Read the model definition and answer for the solid it produces. Units are mm, in the model's axes. Face numbers are marked on the shaded views. A direction names the side the tool comes from. Round coordinates to 2 decimals unless told otherwise and drop trailing zeros. Order: outer loops, then holes, each group sorted by start corner. A loop starts at its lowest first (then second) coordinate and runs counter-clockwise, first axis right, second up. Notation, with made-up numbers: (43, 64.25) - (56, 64.25) arc R16 ccw to (56, 76.25) - close; hole circle Ø8 at (85.25, 3). An arc over 180 degrees is marked (long way). One line per question, with ' | ' between items. Start each with the question number.
1) The part is cut by section A-A, the plane z = 9. Give the vertices of the cut face in (x, y), plus the area to 3 significant figures.
2) Straight lines are drawn through the part: line 1 (Y direction, x = 32, z = 6.5); line 2 (Y direction, x = 38.75, z = 1.05). For each, find the intervals that lie inside material, in ascending order. Write a range as from..to.
3) The part is cut by section C-C, the plane z = 16. Give the vertices of the cut face in (x, y), plus the area to 3 significant figures.
4) For the marked faces 4, 5 and 6, determine the directions among +Z, -Z, +X, -X, +Y, -Y from which every point of the face is accessible in a straight line to the end or side of a thin tool.
5) The part is cut by section D-D, the plane x = 23.3. Give the vertices of the cut face in (y, z).
6) Flat-ended cylindrical pins translate along their axes: pin 1 (1.6 mm diameter, centred on y = 1, z = 13.5, fed in from +X); pin 2 (1.8 mm diameter, centred on x = 38.75, y = 38.75, fed in from +Z); pin 3 (3.5 mm diameter, centred on x = 38.75, y = 7.75, fed in from +Z); pin 4 (2 mm diameter, centred on x = 45.5, z = 13, fed in from +Y). Find the tip coordinate at first contact, or state that the pin passes through.
7) The part is cut by section B-B, the plane y = 23.3. Give the vertices of the cut face in (x, z), plus the area to 3 significant figures.
8) The mould has two halves that part along Y. Classify the marked faces 1, 2 and 3: pulls with the +Y half, pulls with the -Y half, needs draft (parallel to the pull), parting line crosses it, or undercut.
from build123d import *

# Parameters (mm, degrees)
F0_W      = 46.5
F0_H      = 46.5
F0_R      = 1.5
F0_R_2    = 17.5
F1_DEPTH  = 3
F2_W      = 42.5
F2_H      = 2
F3_DEPTH  = 15
F4_W      = 10
F4_H      = 15
F5_DEPTH  = 10
F6_W      = 10
F6_H      = 15
F7_DEPTH  = 10
F8_W      = 10
F8_H      = 15
F9_DEPTH  = 10
F10_W     = 10
F10_H     = 15
F11_DEPTH = 10
F12_R     = 5
F13_R     = 5
F14_R     = 5
F15_R     = 5
F16_W     = 10
F16_H     = 8
F17_DEPTH = 25
F18_R     = 1
F19_R     = 1


with BuildPart() as f1:
    # F0 (on Top) → F1 (new body)
    with BuildSketch(Plane.XY):
        with Locations((23.25, 23.25)):
            Rectangle(F0_W, F0_H)
        with Locations((7.75, 7.75)):
            Circle(F0_R, mode=Mode.SUBTRACT)
        with Locations((38.75, 7.75)):
            Circle(F0_R, mode=Mode.SUBTRACT)
        with Locations((7.75, 38.75)):
            Circle(F0_R, mode=Mode.SUBTRACT)
        with Locations((23.3, 23.3)):
            Circle(F0_R_2, mode=Mode.SUBTRACT)
        with Locations((38.75, 38.75)):
            Circle(F0_R, mode=Mode.SUBTRACT)
    extrude(amount=F1_DEPTH)

    # F2 (on face) → F3 (join)
    with BuildSketch(Plane.XY.offset(3)):
        Polygon((2, 46.5), (0, 46.5), (0, 0), (2, 0), (2, 2), (2, 44.5), align=None)
        with Locations((23.25, 45.5)):
            Rectangle(F2_W, F2_H)
        Polygon((46.5, 46.5), (44.5, 46.5), (44.5, 44.5), (44.5, 2), (44.5, 0), (46.5, 0), align=None)
        with Locations((23.25, 1)):
            Rectangle(F2_W, F2_H)
    extrude(amount=F3_DEPTH)

    # F4 (on face) → F5 (cut)
    with BuildSketch(Plane.XZ):
        with Locations((5, 10.5)):
            Rectangle(F4_W, F4_H)
    extrude(amount=-F5_DEPTH, mode=Mode.SUBTRACT)

    # F6 (on face) → F7 (cut)
    with BuildSketch(Plane(origin=(0, 46.5, 0), x_dir=(-1, 0, 0), z_dir=(0, 1, 0))):
        with Locations((-5, 10.5)):
            Rectangle(F6_W, F6_H)
    extrude(amount=-F7_DEPTH, mode=Mode.SUBTRACT)

    # F8 (on face) → F9 (cut)
    with BuildSketch(Plane(origin=(0, 46.5, 0), x_dir=(-1, 0, 0), z_dir=(0, 1, 0))):
        with Locations((-41.5, 10.5)):
            Rectangle(F8_W, F8_H)
    extrude(amount=-F9_DEPTH, mode=Mode.SUBTRACT)

    # F10 (on face) → F11 (cut)
    with BuildSketch(Plane.XZ):
        with Locations((41.5, 10.5)):
            Rectangle(F10_W, F10_H)
    extrude(amount=-F11_DEPTH, mode=Mode.SUBTRACT)

    # F12
    f12_edges = [f1.edges().sort_by_distance(p)[0] for p in [
        (46.5, 46.5, 1.5),
    ]]
    fillet(f12_edges, radius=F12_R)

    # F13
    f13_edges = [f1.edges().sort_by_distance(p)[0] for p in [
        (0, 46.5, 1.5),
    ]]
    fillet(f13_edges, radius=F13_R)

    # F14
    f14_edges = [f1.edges().sort_by_distance(p)[0] for p in [
        (46.5, 0, 1.5),
    ]]
    fillet(f14_edges, radius=F14_R)

    # F15
    f15_edges = [f1.edges().sort_by_distance(p)[0] for p in [
        (0, 0, 1.5),
    ]]
    fillet(f15_edges, radius=F15_R)

    # F16 (on face) → F17 (cut)
    with BuildSketch(Plane.XZ):
        with Locations((23.25, 14)):
            Rectangle(F16_W, F16_H)
    extrude(amount=-F17_DEPTH, mode=Mode.SUBTRACT)

    # F18
    f18_edges = [f1.edges().sort_by_distance(p)[0] for p in [
        (28.25, 1, 10),
        (18.25, 1, 10),
    ]]
    fillet(f18_edges, radius=F18_R)

    # F19
    f19_edges = [f1.edges().sort_by_distance(p)[0] for p in [
        (18.25, 1, 18),
        (28.25, 1, 18),
    ]]
    fillet(f19_edges, radius=F19_R)


solid = f1.part
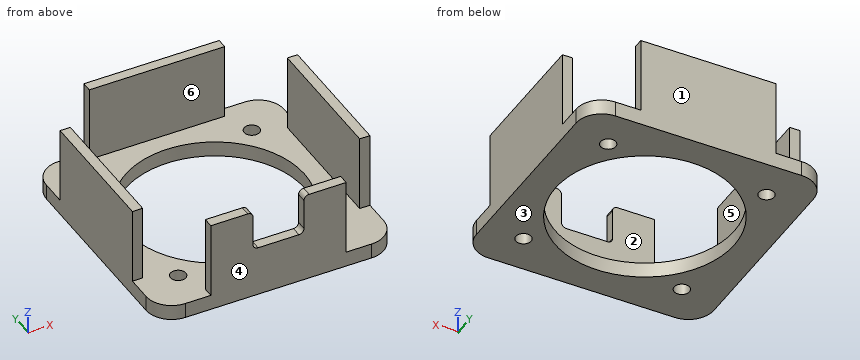
Values:
1) outline: (0, 10) - (2, 10) - (2, 36.5) - (0, 36.5) - close; (10, 0) - (36.5, 0) - (36.5, 2) - (10, 2) - close; (10, 44.5) - (36.5, 44.5) - (36.5, 46.5) - (10, 46.5) - close; (44.5, 10) - (46.5, 10) - (46.5, 36.5) - (44.5, 36.5) - close | area: 212 mm^2
2) line 1: y = 0..2, 44.5..46.5 | line 2: y = 0..6.25, 9.25..15.08, 31.52..37.25, 40.25..46.5
3) outline: (0, 10) - (2, 10) - (2, 36.5) - (0, 36.5) - close; (10, 0) - (18.25, 0) - (18.25, 2) - (10, 2) - close; (10, 44.5) - (36.5, 44.5) - (36.5, 46.5) - (10, 46.5) - close; (28.25, 0) - (36.5, 0) - (36.5, 2) - (28.25, 2) - close; (44.5, 10) - (46.5, 10) - (46.5, 36.5) - (44.5, 36.5) - close | area: 192 mm^2
4) face 4: +Z, -Z, +X, -X, -Y | face 5: +Z, +Y, -Y | face 6: +Z, +X, -X
5) outline: (0, 0) - (5.8, 0) - (5.8, 3) - (2, 3) - (2, 10) - (0, 10) - close; (40.8, 0) - (46.5, 0) - (46.5, 18) - (44.5, 18) - (44.5, 3) - (40.8, 3) - close
6) pin 1: stops at x = 36.5 | pin 2: passes through | pin 3: stops at z = 3 | pin 4: stops at y = 36.5
7) outline: (0, 0) - (5.8, 0) - (5.8, 3) - (2, 3) - (2, 18) - (0, 18) - close; (40.8, 0) - (46.5, 0) - (46.5, 18) - (44.5, 18) - (44.5, 3) - (40.8, 3) - close | area: 94.5 mm^2
8) face 1: pulls with the +Y half | face 2: undercut | face 3: needs draft
